```python
from build123d import *

# Parameters (mm, degrees)
F0_W      = 60
F0_H      = 40
F1_DEPTH  = 2.4
F3_DEPTH  = 1.2
F13_DEPTH = 30
F14_R     = 3
F15_R     = 1


with BuildPart() as f1:
    # F0 (on Top) → F1 (new body)
    with BuildSketch(Plane.XY):
        Rectangle(F0_W, F0_H)
    extrude(amount=-F1_DEPTH)



with BuildPart() as f3:
    # F2 (on Front) → F3 (new body, symmetric)
    with BuildSketch(Plane.XZ):
        Polygon((-30, 30), (-30, 0), (-6, 0), (-20, 30), align=None)
    extrude(amount=F3_DEPTH, both=True)


with BuildPart() as f3b:
    # F2 (on Front) → F3, piece 2 (new body, symmetric)
    with BuildSketch(Plane.XZ):
        Polygon((6, 0), (30, 0), (30, 30), (20, 30), align=None)
    extrude(amount=F3_DEPTH, both=True)


with BuildPart() as f4_1:
    # F4: copy of F3
    add(f3.part.moved(Location((0, 18.8, 0))))


with BuildPart() as f5_1:
    # F5: copy of F3
    add(f3.part.moved(Location((0, -18.8, 0))))


with BuildPart() as f6_1:
    # F6: copy of F3b
    add(f3b.part.moved(Location((0, 18.8, 0))))


with BuildPart() as f7_1:
    # F7: copy of F3b
    add(f3b.part.moved(Location((0, -18.8, 0))))


with BuildPart() as f8_1:
    # F8: copy of F3
    add(f3.part.moved(Location((2.4, 0, 0))))


with BuildPart() as f8_2:
    # F8: copy of F5_1
    add(f5_1.part.moved(Location((2.4, 0, 0))))


with BuildPart() as f8_3:
    # F8: copy of F4_1
    add(f4_1.part.moved(Location((2.4, 0, 0))))


with BuildPart() as f1_1:
    add(f1.part)

    add(f3.part)  # F13 merges F3

    add(f3b.part)  # F13 merges F3b

    add(f4_1.part)  # F13 merges F4_1

    add(f5_1.part)  # F13 merges F5_1

    add(f6_1.part)  # F13 merges F6_1

    add(f7_1.part)  # F13 merges F7_1
    # F12 (on face) → F13 (join)
    with BuildSketch(Plane.XY):
        Polygon((27.6, 17.6), (27.6, -17.6), (27.6, -20), (30, -20), (30, 20), (27.6, 20), align=None)
        Polygon((-27.6, -20), (-27.6, -17.6), (-27.6, 17.6), (-27.6, 20), (-30, 20), (-30, -20), align=None)
    extrude(amount=F13_DEPTH)

    # F14
    f14_edges = [f1_1.edges().sort_by_distance(p)[0] for p in [
        (30, -20, 13.8),
        (-30, -20, 13.8),
        (-30, 20, 13.8),
        (30, 20, 13.8),
    ]]
    fillet(f14_edges, radius=F14_R)

    # F15
    f15_edges = [f1_1.edges().sort_by_distance(p)[0] for p in [
        (20, 18.8, 30),
        (20, 0, 30),
        (20, -18.8, 30),
        (6, 18.8, 0),
        (6, 0, 0),
        (6, -18.8, 0),
        (-20, 18.8, 30),
        (-20, 0, 30),
        (-20, -18.8, 30),
        (-6, -18.8, 0),
        (-6, 0, 0),
        (-6, 18.8, 0),
        (30, 0, 30),
        (-30, 0, 30),
    ]]
    fillet(f15_edges, radius=F15_R)


solid = f1_1.part
```
Model file for the job. Use its own axes, mm. A direction names the side the tool comes from. Round coordinates to 2 decimals unless told otherwise and drop trailing zeros. Loops run counter-clockwise (first coordinate to the right, second up) from the corner with the lowest first, then second, coordinate; pieces in that order, holes last. Notation, with made-up numbers: M 77,49.25 L 127,49.25 A25 cw 127,77.25 Z; hole C 55.5,-8.75 d11. An arc over 180 degrees is marked long. Put each result on its own line as item: value. Start each with the question number.
Item 1: Mould opens along Y. For faces 1 (the face through (29.1, -19.14, 13.08)), 2 (the face through (19, -1.2, 12)), 3 (the face through (-30, 0, 14)), 4 (the face through (-19, 17.6, 12)) say: released by +Y, released by -Y, zero draft, split by the parting line, or undercut.
Item 2: Cut at C-C (x = -25). List the corners of the cut face in (y, z), then the cut area to 3 significant figures.
Item 3: 3-axis set-ups, long thin cutter, end or side, ignore diameter. For faces 5 (the face through (13, 19, 15)), 6 (the face through (-0.4, 20, -0.4)), 7 (the face through (-27.6, 9, 15)): which of +Z, -Z, +X, -X, +Y, -Y reach the whole face in a straight line?
Item 4: Cut at D-D (z = 19.5). List the corners of the cut face in (x, y), then the cut area to 3 significant figures.
Item 5: Cut at A-A (z = 6). List the corners of the cut face in (x, y).
Item 6: Cut at B-B (y = 6.5). List the corners of the cut face in (x, z), then the cut area to 3 significant figures.
Item 7: Drill centre lines: line 1 along Y through (x, z) = (-19.5, 10); line 2 along X through (y, z) = (12, 16); line 3 along Z through (x, y) = (1.5, 11). Where is each one in solid material? Low to high.
Answer block:
1. face 1: released by -Y
1. face 2: undercut
1. face 3: zero draft
1. face 4: undercut
2. outline: M -20,-2.4 L 20,-2.4 L 20,29 A1 ccw 19,30 L 17.6,30 L 17.6,0 L 1.2,0 L 1.2,30 L -1.2,30 L -1.2,0 L -17.6,0 L -17.6,30 L -19,30 A1 ccw -20,29 Z
2. area: 312 mm2
3. face 5: +Z, +Y, -Y
3. face 6: +Z, -Z, +X, -X, +Y
3. face 7: +Z
4. outline: M -30,-17 A3 ccw -27,-20 L -15.1,-20 L -15.1,-17.6 L -27.6,-17.6 L -27.6,-1.2 L -15.1,-1.2 L -15.1,1.2 L -27.6,1.2 L -27.6,17.6 L -15.1,17.6 L -15.1,20 L -27,20 A3 ccw -30,17 Z; M 15.1,-20 L 27,-20 A3 ccw 30,-17 L 30,17 A3 ccw 27,20 L 15.1,20 L 15.1,17.6 L 27.6,17.6 L 27.6,1.2 L 15.1,1.2 L 15.1,-1.2 L 27.6,-1.2 L 27.6,-17.6 L 15.1,-17.6 Z
4. area: 364 mm2
5. outline: M -30,-17 A3 ccw -27,-20 L -8.8,-20 L -8.8,-17.6 L -27.6,-17.6 L -27.6,-1.2 L -8.8,-1.2 L -8.8,1.2 L -27.6,1.2 L -27.6,17.6 L -8.8,17.6 L -8.8,20 L -27,20 A3 ccw -30,17 Z; M 8.8,-20 L 27,-20 A3 ccw 30,-17 L 30,17 A3 ccw 27,20 L 8.8,20 L 8.8,17.6 L 27.6,17.6 L 27.6,1.2 L 8.8,1.2 L 8.8,-1.2 L 27.6,-1.2 L 27.6,-17.6 L 8.8,-17.6 Z
6. outline: M -30,-2.4 L 30,-2.4 L 30,29 A1 ccw 29,30 L 27.6,30 L 27.6,0 L -27.6,0 L -27.6,30 L -29,30 A1 ccw -30,29 Z
6. area: 288 mm2
7. line 1: -20 to -17.6, -1.2 to 1.2, 17.6 to 20
7. line 2: -30 to -27.6, 27.6 to 30
7. line 3: -2.4 to 0
